```python
from build123d import *

# Parameters (mm, degrees)
SKETCH3_W            = 25.753050404
SKETCH3_H            = 103.137359271
BOSS_EXTRUDE1_DEPTH  = 12.7
SKETCH4_R            = 38.1
BOSS_EXTRUDE2_DEPTH  = 25.4
CUT_SWEEP1_PROFILE_R = 7.366


with BuildPart() as part:
    # Sketch3 → Boss-Extrude1 (new body)
    with BuildSketch(Plane(origin=(0, 717.636591226, 0), x_dir=(-1, 0, 0), z_dir=(0, -1, 0))):
        with Locations((-511.2749233, -660.547915429)):
            Rectangle(SKETCH3_W, SKETCH3_H)
    extrude(amount=BOSS_EXTRUDE1_DEPTH)

    # Sketch4 → Boss-Extrude2 (add)
    with BuildSketch(Plane(origin=(524.151448502, 0, 0), x_dir=(0, 0, -1), z_dir=(1, 0, 0))):
        with Locations((-660.547915428, 679.536591226)):
            Circle(SKETCH4_R)
    extrude(amount=-BOSS_EXTRUDE2_DEPTH)

    # Cut-Sweep1: sweep along a path in Sketch5
    with BuildLine(Plane.XY.offset(660.547915428)) as cut_sweep1_path:
        Line((472.45049051, 692.709335123), (547.766548789, 668.191368615))
    # Cut-Sweep1 profile (on start of the path) → Cut-Sweep1 (sweep, cut)
    with BuildSketch(Plane(origin=(472.45049051, 692.709335123, 660.547915428), x_dir=(0.309545628, 0.95088459, 0), z_dir=(0.95088459, -0.309545628, 0))):
        Circle(CUT_SWEEP1_PROFILE_R)
    sweep(path=cut_sweep1_path.line, mode=Mode.SUBTRACT)


solid = part.part
```
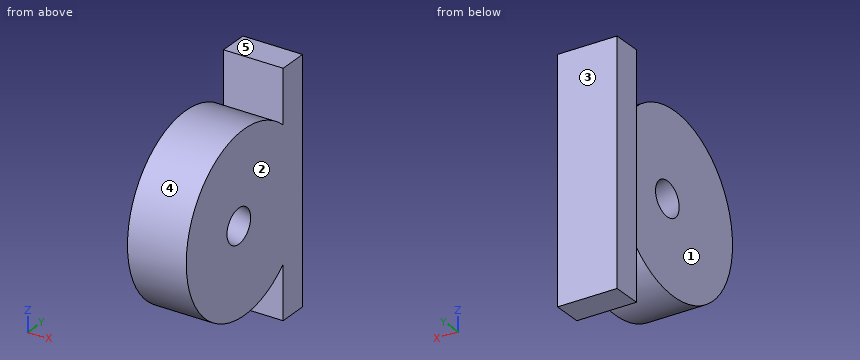
The listing builds one solid part. Answer for the finished solid, in the listing's coordinates (mm). Face numbers are marked on the shaded views. A direction names the side the tool comes from. Coordinates: 2 decimals unless noted, no trailing zeros. Order: outer loops, then holes, each group sorted by start corner. A loop starts at its lowest first (then second) coordinate and runs counter-clockwise, first axis right, second up. Notation, with made-up numbers: M 6.25,18.25 L 42.25,18.25 A12 cw 42.25,38.25 Z; hole C 72,21 d4. An arc over 180 degrees is marked long. Answer as a JSON object with one key per item and string values. Group by question number.
1. Determine the mould class of the marked faces 3, 4 and 5 for opening direction Y: released by +Y, released by -Y, zero draft, split by the parting line, or undercut.
2. Flat-ended cylindrical pins translate along their axes: P1, Ø10, axis at x = 503.5, y = 658.5, coming from the +Z side; P2, Ø6, axis at x = 502.5, y = 684.5, coming from the +Z side; P3, Ø6, axis at y = 695, z = 620, coming from the +X side; P4, Ø1.5, axis at x = 510.5, y = 677, coming from the -Z side. Find the tip coordinate at first contact, or state that the pin passes through.
3. Section C-C on y = 664 is taken. Write down the section's boundary in (x, z), then the cut area to 3 significant figures.
4. A tool of negligible diameter and unlimited length cuts with its end or side. For the marked faces 1 and 2, from which of +Z, -Z, +X, -X, +Y, -Y can it reach the whole face along a straight path? Write none if from no direction.
5. Section A-A on z = 662.5 is taken. Write down the section's boundary in (x, y).
6. Section D-D on z = 675 is taken. Write down the section's boundary in (x, y).
7. Straight lines are drawn through the part: line 1 (Y direction, x = 513, z = 704.5); line 2 (Y direction, x = 521.25, z = 632); line 3 (X direction, y = 700.5, z = 688.5). For each, find the intervals that lie inside material, in ascending order.
8. Section B-B on z = 692.5 is taken. Write down the section's boundary in (x, y).
Values follow:
{
 "1": {"face 3": "released by +Y", "face 4": "undercut", "face 5": "zero draft"},
 "2": {"P1": "z = 695.11", "P2": "z = 698.6", "P3": "through", "P4": "z = 622.49"},
 "3": {"outline": "M 498.75,625.76 L 524.15,625.76 L 524.15,695.34 L 498.75,695.34 Z", "area": "1,770 mm2"},
 "4": {"face 1": "+Z, -Z, -X, -Y", "face 2": "+Z, -Z, +X, +Y, -Y"},
 "5": {"outline": "M 498.4,704.94 L 498.75,704.94 L 498.75,691.62 L 524.15,683.35 L 524.15,717.64 L 498.4,717.64 Z; M 498.75,641.49 L 524.15,641.49 L 524.15,668.41 L 498.75,676.68 Z"},
 "6": {"outline": "M 498.4,704.94 L 498.75,704.94 L 498.75,644.28 L 524.15,644.28 L 524.15,717.64 L 498.4,717.64 Z"},
 "7": {"line 1": "704.94 to 717.64", "line 2": "654.31 to 704.77, 704.94 to 717.64", "line 3": "498.75 to 524.15"},
 "8": {"outline": "M 498.4,704.94 L 524.15,704.94 L 524.15,717.64 L 498.4,717.64 Z; M 498.75,658.78 L 524.15,658.78 L 524.15,700.29 L 498.75,700.29 Z"}
}
